Input: part model. Units: mm. Frame: model coordinates. Face numbers are marked on the shaded views. Round coordinates to 2 decimals unless told otherwise and drop trailing zeros. Loops run counter-clockwise (first coordinate to the right, second up) from the corner with the lowest first, then second, coordinate; pieces in that order, holes last. Notation, with made-up numbers: (23.5, 46.25) - (39.5, 46.25) arc R7 cw to (39.5, 56.25) - close; hole circle Ø8 at (7, 83). An arc over 180 degrees is marked (long way). Write each question's results on one line, items separated by ' | '.
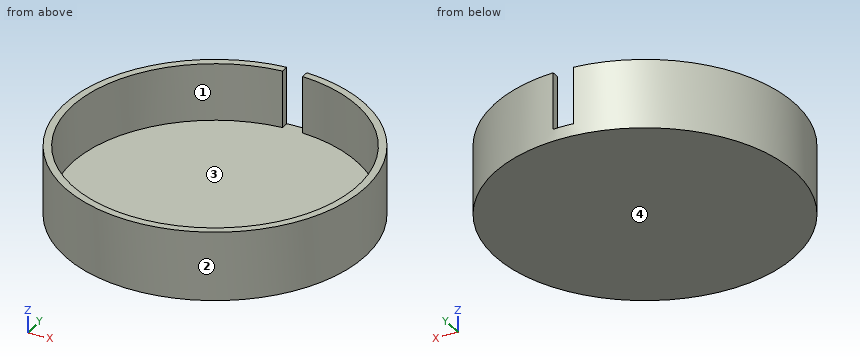
Autodesk Inventor part; units mm, degrees
ref_plane "YZ Plane" through (0, 0, 0) normal (1, 0, 0) x (0, 1, 0)
ref_plane "XZ Plane" through (0, 0, 0) normal (0, 1, 0) x (-1, 0, 0)
ref_plane "XY Plane" through (0, 0, 0) normal (0, 0, 1) x (1, 0, 0)
sketch "Sketch1" plane through (0, 0, 0) normal (0, 0, 1) x (1, 0, 0)
  circle A0 centre (0, 0) radius 25
  dimension "d0" = 50
extrude "Extrusion1" add sketch "Sketch1" along normal blind 11.5
sketch "Sketch2" plane through (0, 0, 11.5) normal (0, 0, 1) x (1, 0, 0)
  arc A0 (-1.6631, 23.6917) -> (1.6631, 23.6917) centre (0, 0) ccw
  line L0 (1.6631, 23.6917) -> (-1.6631, 23.6917)
  dimension "d4" = 47.5
  dimension "d8" = 23.6917
extrude "Extrusion2" cut sketch "Sketch2" against normal blind 9.5
sketch "Sketch3" plane through (-1.6631, 23.6917, 11.5) normal (0, -1, 0) x (1, 0, 0)
  line L0 (0, 0) -> (3.3261, 0)
  line L1 (3.3261, 0) -> (3.3261, -9.5)
  line L2 (3.3261, -9.5) -> (0, -9.5)
  line L3 (0, -9.5) -> (0, 0)
  point P0 (1.6631, -11.5)
  dimension "d9" = 9.5
  dimension "d10" = 3.3261
extrude "Extrusion3" cut sketch "Sketch3" against normal blind 1.5
properties part number "pruebaCargadorReceptor"
1. Mould query, pull axis X, two halves, no side actions, for the marked faces 1, 2, 3 and 4. Classes: pulls with the +X half, pulls with the -X half, needs draft (parallel to the pull), parting line crosses it, or undercut.
Answer:
face 1: undercut | face 2: parting line crosses it | face 3: undercut | face 4: needs draft
2. Section query C-C, the plane x = 0. Output: boundary loops of the cut face in (y, z), plus the area to 3 significant figures.
Answer:
outline: (-25, 0) - (25, 0) - (25, 2) - (-23.75, 2) - (-23.75, 11.5) - (-25, 11.5) - close | area: 112 mm^2
3. Section query B-B, the plane y = 0. Output: boundary loops of the cut face in (x, z).
Answer:
outline: (-25, 0) - (25, 0) - (25, 11.5) - (23.75, 11.5) - (23.75, 2) - (-23.75, 2) - (-23.75, 11.5) - (-25, 11.5) - close
4. Section query D-D, the plane y = 11. Output: boundary loops of the cut face in (x, z), plus the area to 3 significant figures.
Answer:
outline: (-22.45, 0) - (22.45, 0) - (22.45, 11.5) - (21.05, 11.5) - (21.05, 2) - (-21.05, 2) - (-21.05, 11.5) - (-22.45, 11.5) - close | area: 116 mm^2
5. Contact query for flat-ended pins moving along their axis: pin 1 (4 mm diameter, centred on x = -14.5, y = -10.5, fed in from +Z); pin 2 (2 mm diameter, centred on x = -12.5, z = 4, fed in from +Y); pin 3 (1 mm diameter, centred on y = -13.5, z = 5, fed in from +X). Output: stop coordinate, or through.
Answer:
pin 1: z = 2 | pin 2: y = 22.2 | pin 3: x = 21.35
6. Line query: line 1 (X direction, y = 0, z = 4); line 2 (Z direction, x = -4, y = -12); line 3 (X direction, y = -14.5, z = 8.75). Output: solid intervals per line, ascending. Write a range as [from, to].
Answer:
line 1: [-25, -23.75], [23.75, 25] | line 2: [0, 2] | line 3: [-20.37, -18.81], [18.81, 20.37]
